from build123d import *

# Parameters (mm, degrees)
F0_W     = 45
F0_H     = 135
F1_DEPTH = 4
F2_SIZE  = 44.99999
F5_DEPTH = 39.1207225621
F7_D     = 3
F9_D     = 3
F11_D    = 3
F14_D    = 3


# Not quite as in the source:
# - a fillet or chamfer is up to 0.001 mm smaller than in the source, because OpenCascade refuses the exact size


with BuildPart() as f1:
    # F0 (on Top) → F1 (new body)
    with BuildSketch(Plane.XY):
        with Locations((22.5, 67.5)):
            Rectangle(F0_W, F0_H)
    extrude(amount=F1_DEPTH)

    # F2 (size 45 in the source; OpenCascade refuses exactly that, so slightly less here)
    f2_edges = [f1.edges().sort_by_distance(p)[0] for p in [
        (45, 135, 2),
    ]]
    chamfer(f2_edges, length=F2_SIZE)

    # F4 (on face) → F5 (cut)
    with BuildSketch(Plane.XY.offset(4)):
        with BuildLine():
            ThreePointArc((32.5, 20), (35, 17.5), (37.5, 20))
            Line((37.5, 20), (37.5, 70))
            ThreePointArc((37.5, 70), (35, 72.5), (32.5, 70))
            Line((32.5, 70), (32.5, 20))
        make_face()
    extrude(amount=-F5_DEPTH, mode=Mode.SUBTRACT)

    # F7 (through all)
    with Locations(Plane.XY.offset(4)):
        with Locations((16.5778252002, 7.9720381196)):
            Hole(F7_D / 2)

    # F9 (through all)
    with Locations(Plane.XY.offset(4)):
        with Locations((25, 30.5)):
            Hole(F9_D / 2)

    # F11 (through all)
    with Locations(Plane.XY.offset(4)):
        with Locations((25, 54.5)):
            Hole(F11_D / 2)

    # F12: F1 across plane


with BuildPart() as f1_1:
    add(f1.part)
    add(f1.part.mirror(Plane.YZ))

    # F14 (through all)
    with Locations(Plane.XY.offset(4)):
        with Locations((-9.6168344989, 118.5341477394), (8.3831655011, 118.5341477394)):
            Hole(F14_D / 2)


solid = f1_1.part
Here's how the part is built. I have some questions about the finished solid (model axes, mm). A direction names the side the tool comes from. Give positions to 0.01 mm unless a question says otherwise; leave off trailing zeros. Order: outer loops, then holes, each group sorted by start corner. A loop starts at its lowest first (then second) coordinate and runs counter-clockwise, first axis right, second up. Notation, with made-up numbers: M 54,10.5 L 72,10.5 A10 ccw 72,16.5 Z; hole C 54.5,1 d5. An arc over 180 degrees is marked long. Answer as a JSON object with one key per item and string values. Group by question number.
1) Suppose I cut it at D-D, the plane x = -25. Write out the boundary of the cut face in (y, z), plus the area to 3 significant figures.
2) We'd pull the mould along Y, two halves only. Please class faces 1 (the flat face through (1, 0, 2)), 2 (the cylindrical face through (-35.1, 72.5, 2)), 3 (the flat face through (1, 53, 4)): pulls with the +Y half, pulls with the -Y half, needs draft (parallel to the pull), parting line crosses it, or undercut.
3) Suppose I cut it at B-B, the plane x = -35. Write out the boundary of the cut face in (y, z), plus the area to 3 significant figures.
4) Suppose I cut it at C-C, the plane z = 0.6. Count the separate pieces of the cut face and the enclosed holes in it, plus the area to 3 significant figures.
5) On a 3-axis mill with a long thin cutter (end or side, diameter ignored), from which of +Z, -Z, +X, -X, +Y, -Y can I reach the whole of each face in a straight line? I mean faces 4 (the flat face through (22, 113, 2)), 5 (the cylindrical face through (-34.9, 17.5, 2)). Say none if no direction works.
6) Please list where these lines run through material, in increasing order: L1, parallel to X at y = 27.5, z = 1.65; L2, parallel to X at y = 18.5, z = 1.45; L3, parallel to Y at x = 25, z = 2.25. Write a range as [from, to].
7) Suppose I cut it at A-A, the plane y = 62. Write out the boundary of the cut face in (x, z), plus the area to 3 significant figures.
8) I'm going to push a flat-ended pin straight in: pin 1 Ø3 at (x, y) = (24, 24) entering from -Z. Where does the tip first touch, or does it pass through?
Results found:
{
 "1": {"outline": "M 0,0 L 29,0 L 29,4 L 0,4 Z; M 32,0 L 53,0 L 53,4 L 32,4 Z; M 56,0 L 110,0 L 110,4 L 56,4 Z", "area": "416 mm²"},
 "2": {"face 1": "pulls with the -Y half", "face 2": "undercut", "face 3": "needs draft"},
 "3": {"outline": "M 0,0 L 17.5,0 L 17.5,4 L 0,4 Z; M 72.5,0 L 100,0 L 100,4 L 72.5,4 Z", "area": "180 mm²"},
 "4": {"separate pieces": "1", "enclosed holes": "10", "area": "9,530 mm²"},
 "5": {"face 4": "+Z, -Z, +X, +Y", "face 5": "+Z, -Z"},
 "6": {"L1": "[-45, -37.5], [-32.5, 32.5], [37.5, 45]", "L2": "[-45, -37], [-33, 33], [37, 45]", "L3": "[0, 29], [32, 53], [56, 110]"},
 "7": {"outline": "M -45,0 L -37.5,0 L -37.5,4 L -45,4 Z; M -32.5,0 L 32.5,0 L 32.5,4 L -32.5,4 Z; M 37.5,0 L 45,0 L 45,4 L 37.5,4 Z", "area": "320 mm²"},
 "8": {"pin 1": "z = 0"}
}
